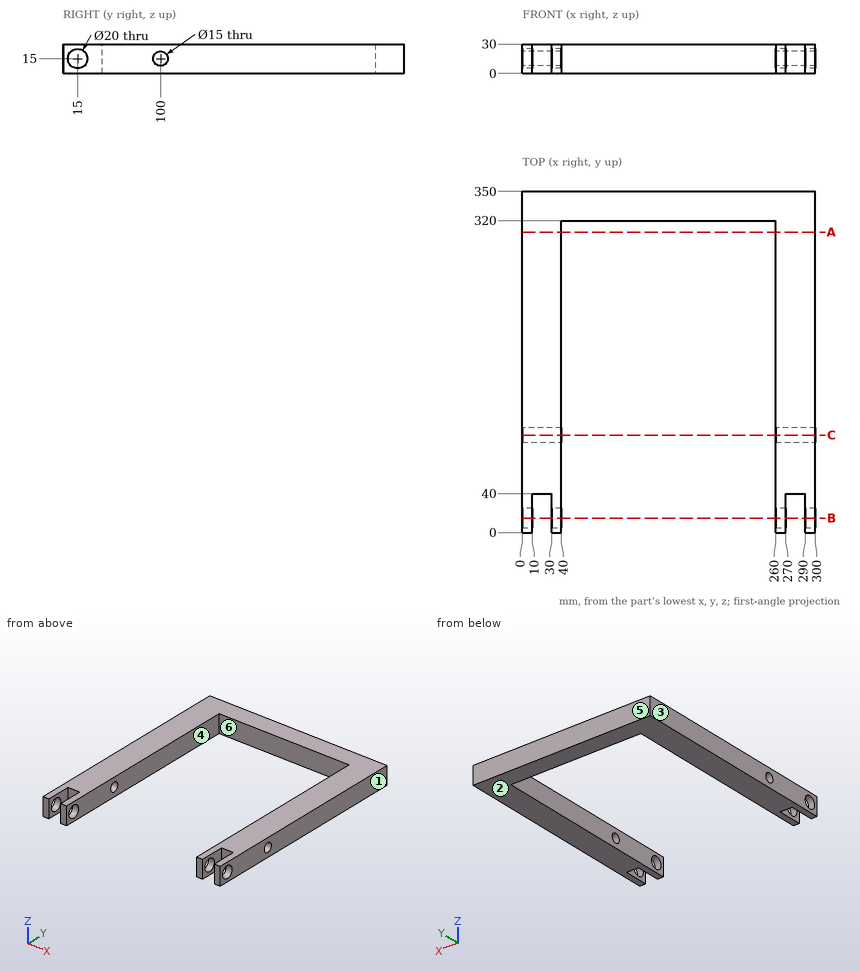
Geometry check sheet. Reference: drawing and pictorial views, mm from the part's lowest x, y, z. A direction names the side the tool comes from. Give positions to 0.01 mm unless a question says otherwise; leave off trailing zeros. Order: outer loops, then holes, each group sorted by start corner. A loop starts at its lowest first (then second) coordinate and runs counter-clockwise, first axis right, second up. Notation, with made-up numbers: (26, 20) - (70, 20) arc R18 ccw to (70, 29) - close; hole circle Ø1 at (19.25, 59). An arc over 180 degrees is marked (long way). Use one line per item in the form item = value.
1) Access from +Z, -Z, +X, -X, +Y, -Y to the whole of each face (thin tool, end or side, straight path). Record for the marked faces 5 and 6.
Working result:
face_5 = +Z, -Z, +X, -X, +Y
face_6 = +Z, -Z, -Y
2) Sectioned sample at C-C (y = 100). Record the boundary of the cut face in (x, z), and give its area (3 significant figures).
Working result:
outline = (0, 0) - (40, 0) - (40, 7.5) - (0, 7.5) - close; (0, 22.5) - (40, 22.5) - (40, 30) - (0, 30) - close; (260, 0) - (300, 0) - (300, 7.5) - (260, 7.5) - close; (260, 22.5) - (300, 22.5) - (300, 30) - (260, 30) - close
area = 1,200 mm^2
3) Draft check along X on the marked faces 1, 2, 3 and 4. Enter one of: released by +X, released by -X, zero draft, split by the parting line, or undercut.
Working result:
face_1 = released by +X
face_2 = zero draft
face_3 = released by -X
face_4 = undercut
4) Material ranges on probe 1 along Y at (x, z) = (266, 15.75); probe 2 along X at (y, z) = (302, 8.75); probe 3 along Z at (x, y) = (263, 15), recorded low to high. Write a range as from..to.
Working result:
probe_1 = 0..5.03, 24.97..92.54, 107.46..350
probe_2 = 0..40, 260..300
probe_3 = 0..5, 25..30
5) Sectioned sample at A-A (y = 308). Record the boundary of the cut face in (x, z), and give its area (3 significant figures).
Working result:
outline = (0, 0) - (40, 0) - (40, 30) - (0, 30) - close; (260, 0) - (300, 0) - (300, 30) - (260, 30) - close
area = 2,400 mm^2
6) Depth check by flat-ended pin: pin 1 Ø9 at (y, z) = (200, 10.5) entering from -X; pin 2 Ø12 at (x, z) = (120.5, 11.5) entering from -Y; pin 3 Ø9 at (y, z) = (100, 15) entering from -X. Enter the tip coordinate at first touch or a pass-through.
Working result:
pin_1 = 0
pin_2 = 320
pin_3 = through
7) Sectioned sample at B-B (y = 15). Count the separate pieces of the cut face and the enclosed holes in it, and give its area (3 significant figures).
Working result:
separate_pieces = 8
enclosed_holes = 0
area = 400 mm^2
